Here's how the part is built. I have some questions about the finished solid (model axes, mm). A direction names the side the tool comes from. Round coordinates to 2 decimals unless told otherwise and drop trailing zeros. Loops run counter-clockwise (first coordinate to the right, second up) from the corner with the lowest first, then second, coordinate; pieces in that order, holes last. Notation, with made-up numbers: (45.5, 28) - (53.5, 28) arc R21 cw to (53.5, 62) - close; hole circle Ø2 at (44, -36.5). An arc over 180 degrees is marked (long way). Answer as a JSON object with one key per item and string values. Group by question number.
1) Which directions (+Z, -Z, +X, -X, +Y, -Y) give clear straight access to the entire face, cutting with the end or side of a thin tool? Please do faces 1 (the face through (130.9, 0.5, -82)), 2 (the face through (-1, 0, -75)), 3 (the face through (1, -8, 67)), 4 (the face through (1, -20, -61)), 5 (the face through (103.5, -20, -1)).
2) I want a section at B-B, the plane z = 26.5. Please give me the cut outline in (x, y), then the cut area to 3 significant figures.
3) If I drill on line 1 along Z through (x, y) = (-36, -25); line 2 along Z through (x, y) = (-74, -3); line 3 along Y through (x, z) = (-102.5, -1.5), over which ranges is the centre line in solid material (lowest first)? Write a range as [from, to].
4) I want a section at A-A, the plane x = 14.5. Please give me the cut outline in (y, z).
5) I want a section at C-C, the plane y = -17.5. Please give me the cut outline in (x, z).
6) Will these pins go through, and if not, where does the flat tip stop? P1, Ø12, axis at y = -15, z = 20.5, coming from the -X side; P2, Ø2, axis at x = -54, y = -2.5, coming from the -Z side; P3, Ø4, axis at x = 48.5, z = 53.5, coming from the +Y side.
7) If we mould it in two halves opening along X, with no side actions, what happens to faces 6 (the face through (-2, 0, -1)), 7 (the face through (-2, 1, 73)), 8 (the face through (-103.5, -20, -1)), 9 (the face through (123.5, -3, 1))? For each: pulls with the +X half, pulls with the -X half, needs draft (parallel to the pull), parting line crosses it, or undercut.
from build123d import *

# Parameters (mm, degrees)
SKETCH1_W           = 266
SKETCH1_H           = 168
BOSS_EXTRUDE1_DEPTH = 1
SKETCH2_W           = 247
SKETCH2_H           = 149
BOSS_EXTRUDE2_DEPTH = 7
BOSS_EXTRUDE3_DEPTH = 103.5
FILLET1_R           = 7
FILLET2_R           = 1
FILLET3_R           = 2.5
SKETCH4_W           = 224
SKETCH4_H           = 126
CUT_EXTRUDE1_DEPTH  = 1


with BuildPart() as part:
    # Sketch1 → Boss-Extrude1 (new body)
    with BuildSketch(Plane(origin=(0, 0, 0), x_dir=(1, 0, 0), z_dir=(0, 1, 0))):
        Rectangle(SKETCH1_W, SKETCH1_H)
    extrude(amount=BOSS_EXTRUDE1_DEPTH)

    # Sketch2 → Boss-Extrude2 (add)
    with BuildSketch(Plane(origin=(0, 0, 0), x_dir=(1, 0, 0), z_dir=(0, 1, 0))):
        Rectangle(SKETCH2_W, SKETCH2_H)
    extrude(amount=-BOSS_EXTRUDE2_DEPTH)

    # Sketch3 → Boss-Extrude3 (add, symmetric)
    with BuildSketch(Plane(origin=(0, 0, 0), x_dir=(0, 0, -1), z_dir=(1, 0, 0))):
        Polygon((-73, -7), (73, -7), (73, -8), (61, -8), (61, -34), (-61, -34), (-61, -8), (-73, -8), align=None)
    extrude(amount=BOSS_EXTRUDE3_DEPTH, both=True)

    # Fillet1
    fillet1_edges = [part.edges().sort_by_distance(p)[0] for p in [
        (-133, 0.5, -84),
        (133, 0.5, -84),
        (133, 0.5, 84),
        (-133, 0.5, 84),
    ]]
    fillet(fillet1_edges, radius=FILLET1_R)

    # Fillet2
    fillet2_edges = [part.edges().sort_by_distance(p)[0] for p in [
        (-123.5, -3.5, 74.5),
        (-123.5, -3.5, -74.5),
        (123.5, -3.5, -74.5),
        (123.5, -3.5, 74.5),
    ]]
    fillet(fillet2_edges, radius=FILLET2_R)

    # Fillet3
    fillet3_edges = [part.edges().sort_by_distance(p)[0] for p in [
        (-103.5, -7.5, 73),
        (0, -34, 61),
        (0, -34, -61),
        (-103.5, -7.5, -73),
        (103.5, -7.5, 73),
        (103.5, -7.5, -73),
    ]]
    fillet(fillet3_edges, radius=FILLET3_R)

    # Sketch4 → Cut-Extrude1 (cut)
    with BuildSketch(Plane(origin=(0, 1, 0), x_dir=(1, 0, 0), z_dir=(0, 1, 0))):
        Rectangle(SKETCH4_W, SKETCH4_H)
    extrude(amount=-CUT_EXTRUDE1_DEPTH, mode=Mode.SUBTRACT)


solid = part.part
Outcome:
{
 "1": {"face 1": "-Z, +X, +Y, -Y", "face 2": "-Y", "face 3": "+Z, +X, -X, -Y", "face 4": "-Z, +X, -X, -Y", "face 5": "+Z, -Z, +X, -Y"},
 "2": {"outline": "(-133, 0) - (-123.5, 0) - (-123.5, -7) - (-103.5, -7) - (-103.5, -34) - (103.5, -34) - (103.5, -7) - (123.5, -7) - (123.5, 0) - (133, 0) - (133, 1) - (112, 1) - (112, 0) - (-112, 0) - (-112, 1) - (-133, 1) - close", "area": "7,360 mm^2"},
 "3": {"line 1": "[-61, 61]", "line 2": "[-74.5, 74.5]", "line 3": "[-34, 0]"},
 "4": {"outline": "(-34, -58.5) arc R2.5 ccw to (-31.5, -61) - (-8, -61) - (-8, -73) - (-7, -73) - (-7, -74.5) - (0, -74.5) - (0, -84) - (1, -84) - (1, -63) - (0, -63) - (0, 63) - (1, 63) - (1, 84) - (0, 84) - (0, 74.5) - (-7, 74.5) - (-7, 73) - (-8, 73) - (-8, 61) - (-31.5, 61) arc R2.5 ccw to (-34, 58.5) - close"},
 "5": {"outline": "(-103.5, -61) - (103.5, -61) - (103.5, 61) - (-103.5, 61) - close"},
 "6": {"P1": "x = -103.5", "P2": "z = -74.5", "P3": "y = 0"},
 "7": {"face 6": "undercut", "face 7": "needs draft", "face 8": "pulls with the -X half", "face 9": "pulls with the +X half"}
}
